from build123d import *

# Parameters (mm, degrees)
AUFSATZ_LINEAR_AUSTRAGEN1_DEPTH = 165.5
SKIZZE3_R                       = 3.25
SCHNITT_LINEAR_AUSTRAGEN1_DEPTH = 20


with BuildPart() as part:
    # Skizze1 → Aufsatz-Linear austragen1 (new body)
    with BuildSketch(Plane.XY):
        Polygon((-36, 1.5), (36, 1.5), (36, 0), (55, 0), (55, 11.5), (40, 11.5), (40, 73), (-40, 73), (-40, 11.5), (-55, 11.5), (-55, 0), (-36, 0), align=None)
    extrude(amount=AUFSATZ_LINEAR_AUSTRAGEN1_DEPTH)

    # Skizze2 → Rotation1 (revolve)
    with BuildSketch(Plane(origin=(0, 0, 0), x_dir=(0, 0, -1), z_dir=(1, 0, 0))):
        with BuildLine():
            Line((-165.5, 72), (-189.378953192, 67.735901216))
            ThreePointArc((-189.378953192, 67.735901216), (-192.333716602, 66.023532336), (-193.5, 62.813763338))
            Line((-193.5, 62.813763338), (-193.5, 37))
            Line((-193.5, 37), (-165.5, 37))
            Line((-165.5, 37), (-165.5, 72))
        make_face()
        Polygon((0, 72), (11, 72), (11, 68), (33, 68), (33, 62), (35, 62), (36, 61.422649731), (36, 48.6), (51, 48.6), (51, 52.5), (67, 52.5), (67, 37), (0, 37), align=None)
    revolve(axis=Axis((0, 37, -51.73091969), (0, 0, 1)))

    # Skizze3 → Schnitt-Linear austragen1 (cut)
    with BuildSketch(Plane.XZ):
        with Locations((47.5, 30)):
            Circle(SKIZZE3_R)
        with Locations((47.5, 65)):
            Circle(SKIZZE3_R)
        with Locations((47.5, 100)):
            Circle(SKIZZE3_R)
        with Locations((47.5, 135)):
            Circle(SKIZZE3_R)
        with Locations((-47.5, 30)):
            Circle(SKIZZE3_R)
        with Locations((-47.5, 65)):
            Circle(SKIZZE3_R)
        with Locations((-47.5, 100)):
            Circle(SKIZZE3_R)
        with Locations((-47.5, 135)):
            Circle(SKIZZE3_R)
    extrude(amount=-SCHNITT_LINEAR_AUSTRAGEN1_DEPTH, mode=Mode.SUBTRACT)


solid = part.part
For this review, take the finished solid that the model builds, in its own axes (mm). A direction names the side the tool comes from. Coordinates: 2 decimals unless noted, no trailing zeros. Loops run counter-clockwise (first coordinate to the right, second up) from the corner with the lowest first, then second, coordinate; pieces in that order, holes last. Notation, with made-up numbers: (65, 25.25) -> (85, 25.25) arc R16 cw to (85, 42.25) -> close; hole circle Ø4 at (64, 2.5). An arc over 180 degrees is marked (long way). Write each question's results on one line, items separated by ' | '.
Q1. Add section B-B, the plane z = 30. State the section outline as (x, y) points.
Taken from the geometry:
outline: (-55, 0) -> (-50.75, 0) -> (-50.75, 11.5) -> (-55, 11.5) -> close; (-44.25, 0) -> (-36, 0) -> (-36, 1.5) -> (36, 1.5) -> (36, 0) -> (44.25, 0) -> (44.25, 11.5) -> (40, 11.5) -> (40, 73) -> (-40, 73) -> (-40, 11.5) -> (-44.25, 11.5) -> close; (50.75, 0) -> (55, 0) -> (55, 11.5) -> (50.75, 11.5) -> close
Q2. Mouldability with a two-part tool opening along X and no side actions: class faces 6 (the cylindrical face through (49, 5.67, 97.117)), 7 (the cylindrical face through (-7.509, 60.846, -34.014)), 8 (the flat face through (16, 4, 0)) as +X half, -X half, draft (parallel to the pull), parting line (faces both ways), or undercut.
Taken from the geometry:
face 6: undercut | face 7: parting line | face 8: draft
Q3. Machinability: for faces 1 (the flat face through (48, 11.5, 82)), 2 (the flat face through (16, 4, 165.5)), 3 (the flat face through (-47, 11.5, 82)), 4 (the cylindrical face through (-1.36, 6.03, -22.15)), 5 (the cylindrical face through (-0.51, 25.41, -43.6)), which of the approach directions +Z, -Z, +X, -X, +Y, -Y give a long, thin tool a straight path to every point of the face, cutting with its end or side? Answer none if there is none.
Taken from the geometry:
face 1: +Z, -Z, +X, +Y | face 2: +Z | face 3: +Z, -Z, -X, +Y | face 4: -Z | face 5: none
Q4. Add section C-C, the plane z = 86. State the section outline as (x, y) points.
Taken from the geometry:
outline: (-55, 0) -> (-36, 0) -> (-36, 1.5) -> (36, 1.5) -> (36, 0) -> (55, 0) -> (55, 11.5) -> (40, 11.5) -> (40, 73) -> (-40, 73) -> (-40, 11.5) -> (-55, 11.5) -> close
Q5. For pin 1 Ø4 at (x, z) = (47.5, 100) entering from +Y; pin 2 Ø12 at (x, y) = (-15.5, 12) entering from -Z; pin 3 Ø3 at (y, z) = (64, 15.5) entering from -X; pin 4 Ø10 at (x, y) = (40, 34) entering from -Z, all flat-tipped, find the tip position at first contact; note any pin that passes through.
Taken from the geometry:
pin 1: through | pin 2: z = -36 | pin 3: x = -40 | pin 4: z = 0
Q6. To check wall thickness, follow line 1 along Z through (x, y) = (-47.5, 8); line 2 along X through (y, z) = (5.5, 135); line 3 along Z through (x, y) = (-12, 36.5). State the ranges of each line that lie inside material, in increasing order. Write a range as [from, to].
Taken from the geometry:
line 1: [0, 26.75], [33.25, 61.75], [68.25, 96.75], [103.25, 131.75], [138.25, 165.5] | line 2: [-55, -50.75], [-44.25, 44.25], [50.75, 55] | line 3: [-67, -51], [-36, 193.5]
Q7. Add section A-A, the plane x = 47.5. State the section outline as (y, z) points, then the cut area to 3 significant figures.
Taken from the geometry:
outline: (0, 0) -> (11.5, 0) -> (11.5, 26.75) -> (0, 26.75) -> close; (0, 33.25) -> (11.5, 33.25) -> (11.5, 61.75) -> (0, 61.75) -> close; (0, 68.25) -> (11.5, 68.25) -> (11.5, 96.75) -> (0, 96.75) -> close; (0, 103.25) -> (11.5, 103.25) -> (11.5, 131.75) -> (0, 131.75) -> close; (0, 138.25) -> (11.5, 138.25) -> (11.5, 165.5) -> (0, 165.5) -> close | area: 1,600 mm²
